```python
from build123d import *

# Parameters (mm, degrees)
F1_DEPTH     = 10.25
F3_DEPTH     = 2.5
F4_R         = 1
F5_T         = 1.9
F5_T3_DEPTH  = 4.8
F5_T5_DEPTH  = 31.8
F5_T8_ANGLE  = 90.000000001
F5_T10_ANGLE = 90.000000001
F6_R         = 5.5
F7_DEPTH     = 2


# Not quite as in the source:
# - a shell that OpenCascade refuses in one call is made with other operations: the cavity is built on its own and cut out


with BuildPart() as f1:
    # F0 (on Top) → F1 (new body)
    with BuildSketch(Plane.XY):
        with BuildLine():
            Line((16, 19), (-16, 19))
            ThreePointArc((-16, 19), (-21.6568542495, 16.6568542495), (-24, 11))
            Line((-24, 11), (-24, -11))
            ThreePointArc((-24, -11), (-21.6568542495, -16.6568542495), (-16, -19))
            Line((-16, -19), (16, -19))
            ThreePointArc((16, -19), (21.6568542495, -16.6568542495), (24, -11))
            Line((24, -11), (24, 11))
            ThreePointArc((24, 11), (21.6568542495, 16.6568542495), (16, 19))
        make_face()
    extrude(amount=F1_DEPTH)

    # F2 (on face) → F3 (join)
    with BuildSketch(Plane.XY.offset(10.25)):
        with BuildLine():
            Line((12, 21.85), (-16, 21.85))
            ThreePointArc((-16, 21.85), (-21.6568542495, 19.5068542495), (-24, 13.85))
            Line((-24, 13.85), (-24, 11))
            ThreePointArc((-24, 11), (-21.6568542495, 16.6568542495), (-16, 19))
            Line((-16, 19), (12, 19))
            Line((12, 19), (12, 21.85))
        make_face()
        with BuildLine():
            Line((12, -21.85), (12, -19))
            Line((12, -19), (-16, -19))
            ThreePointArc((-16, -19), (-21.6568542495, -16.6568542495), (-24, -11))
            Line((-24, -11), (-24, -13.85))
            ThreePointArc((-24, -13.85), (-21.6568542495, -19.5068542495), (-16, -21.85))
            Line((-16, -21.85), (12, -21.85))
        make_face()
    extrude(amount=-F3_DEPTH)

    # F4
    f4_edges = [f1.edges().sort_by_distance(p)[0] for p in [
        (12, -21.85, 9),
        (12, -19, 9),
        (12, 19, 9),
        (12, 21.85, 9),
    ]]
    fillet(f4_edges, radius=F4_R)

    # F5: shell of thickness 1.9, made by hand


with BuildPart() as f5_core1:
    # F5_t2: copy of F1
    add(f1.part)

    # the walls: a layer under each face that stays
    f5_faces = [f5_core1.faces().sort_by_distance(p)[0] for p in [
        (0, 19, 5.125),
        (0, 0, 10.25),
        (12.2928932188, 19.2928932188, 9),
        (21.6568542495, 16.6568542495, 5.125),
        (-17.8333333333, 20.0416666667, 7.75),
        (-21.6568542495, 16.6568542495, 3.875),
        (12, 20.425, 9),
        (24, 0, 5.125),
        (21.6568542495, -16.6568542495, 5.125),
        (-2.5, 21.85, 9),
        (0, -19, 5.125),
        (-21.6568542495, 19.5068542495, 9),
        (12.2928932188, -19.2928932188, 9),
        (-24, 0, 5.125),
        (12, -20.425, 9),
        (-21.6568542495, -19.5068542495, 9),
        (-2.5, -21.85, 9),
        (-21.6568542495, -16.6568542495, 3.875),
        (-17.8333333333, -20.0416666667, 7.75),
    ]]
    thicken(f5_faces, amount=-F5_T, mode=Mode.SUBTRACT)

    # F5_s4 → F5_t3 (cut)
    with BuildSketch(Plane.YZ.offset(10.1)):
        Polygon((19.019, 7.731), (17.1, 7.75), (17.1, 9.65), (19, 9.65), align=None)
        Polygon((-19.019, 7.731), (-17.1, 7.75), (-17.1, 9.65), (-19, 9.65), align=None)
    extrude(amount=F5_T3_DEPTH, mode=Mode.SUBTRACT)

    # F5_s6 → F5_t5 (cut)
    with BuildSketch(Plane.YZ.offset(-17.9)):
        Polygon((19.019, 7.731), (17.1, 7.75), (17.1, 9.65), (19, 9.65), align=None)
        Polygon((-19.019, 7.731), (-17.1, 7.75), (-17.1, 9.65), (-19, 9.65), align=None)
    extrude(amount=F5_T5_DEPTH, mode=Mode.SUBTRACT)

    # F5_s7 → F5_t8 (revolve, cut)
    with BuildSketch(Plane.XZ.offset(-11)):
        Polygon((-24.019, 7.731), (-24, 9.65), (-22.1, 9.65), (-22.1, 7.75), align=None)
    revolve(axis=Axis((-16, 11, 7.75), (0, 0, -1)), revolution_arc=F5_T8_ANGLE, mode=Mode.SUBTRACT)

    # F5_s9 → F5_t10 (revolve, cut)
    with BuildSketch(Plane.YZ.offset(-16)):
        Polygon((-19.019, 7.731), (-17.1, 7.75), (-17.1, 9.65), (-19, 9.65), align=None)
    revolve(axis=Axis((-16, -11, 7.75), (0, 0, -1)), revolution_arc=F5_T10_ANGLE, mode=Mode.SUBTRACT)


with BuildPart() as f1_1:
    add(f1.part)

    # what is left inside the walls is the cavity
    f5_cavity = [f5_core1.part.solids().sort_by_distance(p)[0] for p in [
        (0, -5.7, 8.331),
    ]]
    add(f5_cavity, mode=Mode.SUBTRACT)

    # F6 (on face) → F7 (cut)
    with BuildSketch(Plane(origin=(-24, 0, 0), x_dir=(0, -1, 0), z_dir=(-1, 0, 0))):
        Circle(F6_R)
    extrude(amount=-F7_DEPTH, mode=Mode.SUBTRACT)


solid = f1_1.part
```
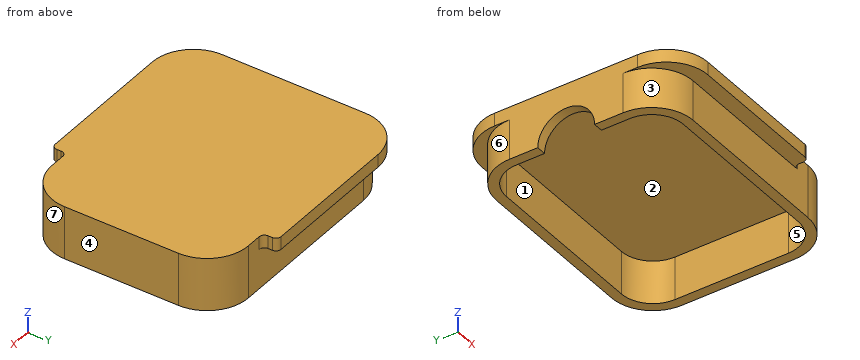
Geometry check sheet. Reference: the model listing, model coordinates, mm. Face numbers are marked on the shaded views. A direction names the side the tool comes from. Round coordinates to 2 decimals unless told otherwise and drop trailing zeros. Loops run counter-clockwise (first coordinate to the right, second up) from the corner with the lowest first, then second, coordinate; pieces in that order, holes last. Notation, with made-up numbers: (-12, 12.25) -> (19, 12.25) arc R24 ccw to (19, 41.25) -> close; hole circle Ø5 at (37, 35). An arc over 180 degrees is marked (long way). Use a Markdown table: item, result.
(1) Scan lines: probe 1 along Y at (x, z) = (2.5, 6.5); probe 2 along Z at (x, y) = (-14.5, 15.5); probe 3 along X at (y, z) = (1.5, 6). Record each from-to range of solid material in increasing order.
Calculated:
| item | result |
|---|---|
| probe 1 | -19 to -17.1, 17.1 to 19 |
| probe 2 | 8.35 to 10.25 |
| probe 3 | -24 to -22.1, 22.1 to 24 |
(2) Go/stop test with flat-tipped pins: P1, Ø0.7, axis at y = 20.5, z = 8.5, coming from the +X side; P2, Ø5, axis at y = 16, z = 4.5, coming from the +X side; P3, Ø4, axis at x = 2.5, z = 2.5, coming from the +Y side. Record where each tip stops, or that it passes through.
Calculated:
| item | result |
|---|---|
| P1 | x = 12 |
| P2 | x = 23.6 |
| P3 | y = 19 |
(3) Sectioned sample at B-B (y = 10). Enter the section's corners in (x, z), then the cut area to 3 significant figures.
Calculated:
| item | result |
|---|---|
| outline | (-24, 0) -> (-22.1, 0) -> (-22.1, 8.35) -> (22.1, 8.35) -> (22.1, 0) -> (24, 0) -> (24, 10.25) -> (-24, 10.25) -> close |
| area | 123 mm² |
(4) Set-up check for the marked faces 5, 6 and 7: record each of +Z, -Z, +X, -X, +Y, -Y from which the full face is reachable in a straight line by a thin tool's end or side.
Calculated:
| item | result |
|---|---|
| face 5 | -Z |
| face 6 | -Z, -X, +Y |
| face 7 | +Z, -Z, +X, -Y |
(5) Mould release check, pull along X, two halves, no side actions. Record for the marked faces 1, 2, 3 and 4: released by +X, released by -X, zero draft, split by the parting line, or undercut.
Calculated:
| item | result |
|---|---|
| face 1 | undercut |
| face 2 | undercut |
| face 3 | released by -X |
| face 4 | released by +X |
(6) Sectioned sample at D-D (y = 0). Enter the section's corners in (x, z), then the cut area to 3 significant figures.
Calculated:
| item | result |
|---|---|
| outline | (-24, 5.5) -> (-22.1, 5.5) -> (-22.1, 8.35) -> (22.1, 8.35) -> (22.1, 0) -> (24, 0) -> (24, 10.25) -> (-24, 10.25) -> close |
| area | 112 mm² |
(7) Sectioned sample at A-A (z = 6.5). Enter the section's corners in (x, y), then the cut area to 3 significant figures.
Calculated:
| item | result |
|---|---|
| outline | (-24, -11) arc R8 ccw to (-16, -19) -> (16, -19) arc R8 ccw to (24, -11) -> (24, 11) arc R8 ccw to (16, 19) -> (-16, 19) arc R8 ccw to (-24, 11) -> close; hole (-22.1, -11) arc R6.1 ccw to (-16, -17.1) -> (16, -17.1) arc R6.1 ccw to (22.1, -11) -> (22.1, 11) arc R6.1 ccw to (16, 17.1) -> (-16, 17.1) arc R6.1 ccw to (-22.1, 11) -> close |
| area | 289 mm² |
(8) Sectioned sample at C-C (x = -8.5). Enter the section's corners in (y, z), then the cut area to 3 significant figures.
Calculated:
| item | result |
|---|---|
| outline | (-21.85, 7.75) -> (-19, 7.75) -> (-19, 0) -> (-17.1, 0) -> (-17.1, 8.35) -> (17.1, 8.35) -> (17.1, 0) -> (19, 0) -> (19, 7.75) -> (21.85, 7.75) -> (21.85, 10.25) -> (-21.85, 10.25) -> close |
| area | 118 mm² |
